The model under review builds one solid part; all positions refer to its coordinate system, in mm. Face numbers are marked on the shaded views. Coordinates: 2 decimals unless noted, no trailing zeros. Loops run counter-clockwise (first coordinate to the right, second up) from the corner with the lowest first, then second, coordinate; pieces in that order, holes last. Notation, with made-up numbers: M -31.5,38.5 L 13.5,38.5 A20 cw 13.5,54.5 Z; hole C 83,15 d9. An arc over 180 degrees is marked long. Use CSV: the item, a comma, the result in double quotes. Start each with the question number.
1. Add section A-A, the plane x = -20. Write out the cut boundary in (y, z), then the cut area to 3 significant figures.
2. Draft analysis for pull direction X (two halves, no side actions). For the marked faces 1, 2, 3 and 4, state which applies: +X half, -X half, draft (parallel to the pull), parting line (faces both ways), or undercut.
3. Add section D-D, the plane x = -46. Write out the cut boundary in (y, z).
4. Clearance check with flat-ended pins moving along their axes: P1, Ø1.5, axis at x = -2.5, y = -39, coming from the -Z side; P2, Ø12, axis at x = -47.5, y = -28.5, coming from the -Z side; P3, Ø2, axis at x = -35, y = -10, coming from the -Z side. State where each tip first meets the part, or that it passes through.
5. Add section C-C, the plane y = -26. Write out the cut boundary in (x, z).
6. Add section B-B, the plane z = -28. Write out the cut boundary in (x, y), then the cut area to 3 significant figures.
7. For L1, parallel to Z at x = -3, y = -48; L2, parallel to Z at x = -11, y = -5.5; L3, parallel to X at y = -46, z = 37.5, list the stretches that pass through material, from the lowest coordinate up.
from build123d import *

# Parameters (mm, degrees)
F0_R     = 74.972812
F1_DEPTH = 50.8
F3_DEPTH = 76.2


with BuildPart() as f1:
    # F0 (on Front) → F1 (new body)
    with BuildSketch(Plane.XZ):
        Circle(F0_R)
    extrude(amount=F1_DEPTH)

    # F2 (on face) → F3 (cut)
    with BuildSketch(Plane.XZ.offset(50.8)):
        Polygon((17.951952, 23.678008), (30.332614, 59.272397), (5.571298, 33.273019), (9.883918, 29.165761), (-5.794326, 12.703607), (0, 7.185201), (-26.807584, -20.962759), (-23.24244, -24.358134), (-42.689349, -44.777386), (4.333233, -14.082998), (0, -9.956109), (21.580685, 12.703607), align=None)
    extrude(amount=-F3_DEPTH, mode=Mode.SUBTRACT)


solid = f1.part
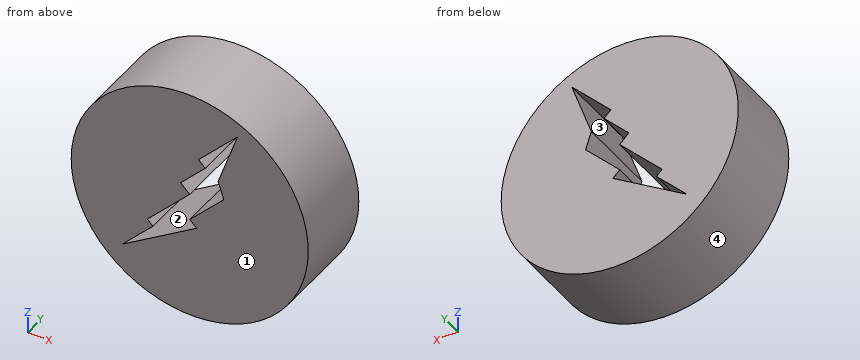
Computed:
1,outline,"M -50.8,-72.26 L 0,-72.26 L 0,-29.97 L -50.8,-29.97 Z; M -50.8,-13.81 L 0,-13.81 L 0,72.26 L -50.8,72.26 Z"
1,area,"6,520 mm^2"
2,face 1,"draft"
2,face 2,"undercut"
2,face 3,"undercut"
2,face 4,"parting line"
3,outline,"M -50.8,-59.2 L 0,-59.2 L 0,59.2 L -50.8,59.2 Z"
4,P1,"stops at z = -74.95"
4,P2,"stops at z = -62.44"
4,P3,"stops at z = -66.82"
5,outline,"C 0,0 d149.95; hole M -42.69,-44.78 L 4.33,-14.08 L 0,-9.96 L 21.58,12.7 L 17.95,23.68 L 30.33,59.27 L 5.57,33.27 L 9.88,29.17 L -5.79,12.7 L 0,7.19 L -26.81,-20.96 L -23.24,-24.36 Z"
6,outline,"M -69.55,-50.8 L -26.71,-50.8 L -26.71,0 L -69.55,0 Z; M -16.99,-50.8 L 69.55,-50.8 L 69.55,0 L -16.99,0 Z"
6,area,"6,570 mm^2"
7,L1,"z = -74.91 to -18.87, 4.04 to 10.04, 15.64 to 74.91"
7,L2,"z = -74.16 to -24.09, -4.36 to 74.16"
7,L3,"x = -64.92 to 9.6, 22.76 to 64.92"
